Design review of the part built by this model. Coordinates are the model's own, in mm. A direction names the side the tool comes from. Give positions to 0.01 mm unless a question says otherwise; leave off trailing zeros. Order: outer loops, then holes, each group sorted by start corner. A loop starts at its lowest first (then second) coordinate and runs counter-clockwise, first axis right, second up. Notation, with made-up numbers: (-19, 10.25) -> (11, 10.25) arc R30 cw to (11, 48.25) -> close; hole circle Ø4 at (33, 60.25). An arc over 180 degrees is marked (long way). One line per item, written item: value.
from build123d import *

# Parameters (mm, degrees)
BOX_W             = 10
BOX_H             = 15
BOX_DEPTH         = 15
PAD_DEPTH         = 2
PAD_DEPTH_BACK    = 7.5
POCKET_DEPTH      = 6.4
POCKET001_DEPTH   = 2.5
PAD005_DEPTH      = 0.45
PAD005_DEPTH_BACK = 0.45
FILLET_R          = 0.5
FILLET008_R       = 0.2
FILLET009_R       = 0.2
FILLET010_R       = 0.5
SKETCH013_W       = 3
SKETCH013_H       = 1
PAD008_DEPTH      = 1
FILLET015_R       = 0.5
FILLET016_R       = 0.99


with BuildPart() as obj1:
    # Box → Box (new body)
    with BuildSketch(Plane(origin=(0, -9, 0), x_dir=(1, 0, 0), z_dir=(0, 0, 1))):
        with Locations((5, 7.5)):
            Rectangle(BOX_W, BOX_H)
    extrude(amount=BOX_DEPTH)


with BuildPart() as obj2:
    # Sketch (on DatumPlane) → Pad (new body, two sides)
    with BuildSketch(Plane.XY.offset(10)) as pad_sk:
        with BuildLine():
            ThreePointArc((5.5, 1.920538), (0, 2.6), (-5.5, 1.920538))
            Line((-5.5, 1.920538), (-3.616372, -5.586761))
            ThreePointArc((3.616372, -5.586761), (0, -5.14), (-3.616372, -5.586761))
            Line((3.616372, -5.586761), (5.5, 1.920538))
        make_face()
    extrude(amount=PAD_DEPTH)
    extrude(pad_sk.sketch, amount=-PAD_DEPTH_BACK)

    # Sketch001 (on Face5 of Pad) → Pocket (cut)
    with BuildSketch(Plane(origin=(0, 0, 2.5), x_dir=(1, 0, 0), z_dir=(0, 0, -1))):
        with BuildLine():
            ThreePointArc((-4.515394, -1.283614), (0, -1.8), (4.515394, -1.283614))
            Line((3.020793, 4.673197), (4.515394, -1.283614))
            ThreePointArc((-3.020793, 4.673197), (0, 4.34), (3.020793, 4.673197))
            Line((-4.515394, -1.283614), (-3.020793, 4.673197))
        make_face()
    extrude(amount=-POCKET_DEPTH, mode=Mode.SUBTRACT)

    # Sketch002 (on Face5 of Pocket) → Pocket001 (cut)
    with BuildSketch(Plane.XY.offset(12)):
        with BuildLine():
            ThreePointArc((4.283186, -2.929138), (0, -2.4), (-4.283186, -2.929138))
            Line((-4.283186, -2.929138), (-3.616372, -5.586761))
            ThreePointArc((3.616372, -5.586761), (0, -5.14), (-3.616372, -5.586761))
            Line((4.283186, -2.929138), (3.616372, -5.586761))
        make_face()
    extrude(amount=-POCKET001_DEPTH, mode=Mode.SUBTRACT)

    # Sketch008 (on DatumPlane) → Pad005 (join, two sides)
    with BuildSketch(Plane.XY.offset(7.95)) as pad005_sk:
        Polygon((-3.9, 2.260952), (-3.9, 4.3), (-3, 4.3), (-2.1, 4.3), (-2.1, 2.502222), align=None)
        Polygon((2.1, 2.502222), (2.1, 4.3), (3, 4.3), (3.9, 4.3), (3.9, 2.260952), align=None)
    extrude(amount=PAD005_DEPTH)
    extrude(pad005_sk.sketch, amount=-PAD005_DEPTH_BACK)

    # Fillet
    fillet_edges = [obj2.edges().sort_by_distance(p)[0] for p in [
        (0, -2.4, 12),
        (4.891593, -0.5043, 12),
        (0, 2.6, 12),
        (-4.891593, -0.5043, 12),
        (4.283186, -2.929138, 10.75),
        (5.5, 1.920538, 7.25),
        (-5.5, 1.920538, 7.25),
        (-4.283186, -2.929138, 10.75),
    ]]
    fillet(fillet_edges, radius=FILLET_R)

    # Fillet008
    fillet008_edges = [obj2.edges().sort_by_distance(p)[0] for p in [
        (-3.616372, -5.586761, 6),
        (3.616372, -5.586761, 6),
        (-4.496657, -2.078339, 2.5),
        (4.496657, -2.078339, 2.5),
    ]]
    fillet(fillet008_edges, radius=FILLET008_R)

    # Fillet009
    fillet009_edges = [obj2.edges().sort_by_distance(p)[0] for p in [
        (0, -4.34, 8.9),
        (-3.768094, -1.694791, 8.9),
        (0, 1.8, 8.9),
        (3.768094, -1.694791, 8.9),
        (4.515394, 1.283614, 5.7),
        (3.020793, -4.673197, 5.7),
        (-3.020793, -4.673197, 5.7),
        (-4.515394, 1.283614, 5.7),
    ]]
    fillet(fillet009_edges, radius=FILLET009_R)

    # Fillet010
    fillet010_edges = [obj2.edges().sort_by_distance(p)[0] for p in [
        (-3.002424, 2.399675, 8.4),
        (-3.002424, 2.399675, 7.5),
        (3.002424, 2.399675, 7.5),
        (3.002424, 2.399675, 8.4),
    ]]
    fillet(fillet010_edges, radius=FILLET010_R)

    # Sketch013 (on Face21 of Fillet010) → Pad008 (join)
    with BuildSketch(Plane(origin=(0, 0, 2.5), x_dir=(1, 0, 0), z_dir=(0, 0, -1))):
        with Locations((0, 3.921408)):
            Rectangle(SKETCH013_W, SKETCH013_H)
    extrude(amount=-PAD008_DEPTH)

    # Fillet015
    fillet015_edges = [obj2.edges().sort_by_distance(p)[0] for p in [
        (0, -4.34, 3.5),
    ]]
    fillet(fillet015_edges, radius=FILLET015_R)

    # Fillet016
    fillet016_edges = [obj2.edges().sort_by_distance(p)[0] for p in [
        (0, -3.421408, 3.5),
    ]]
    fillet(fillet016_edges, radius=FILLET016_R)

    # Cut: cut obj1
    add(obj1.part, mode=Mode.SUBTRACT)


solid = obj2.part
Item 1: Add section C-C on z = 10. Give the boundary of the cut face in (x, y), plus the area to 3 significant figures.
Returned:
outline: (-5.38, 1.43) -> (-4.4, -2.45) arc R0.5 ccw to (-3.81, -2.82) arc R17.6 cw to (0, -2.4) -> (0, 2.6) arc R22.6 ccw to (-5, 2.04) arc R0.5 ccw to start
area: 24.6 mm²
Item 2: Machinability: for faces 1 (the cylindrical face through (-1.444, -4.415, 5.557)), 2 (the cylindrical face through (-2.2, 1.68, 5.56)), 3 (the cylindrical face through (-4.737, -0.501, 11.857)), 4 (the flat face through (-3.9, 3, 8)), which of the approach directions +Z, -Z, +X, -X, +Y, -Y give a long, thin tool a straight path to every point of the face, cutting with its end or side? Answer none if there is none.
Returned:
face 1: none
face 2: -Z, +X
face 3: +Z, -X, -Y
face 4: +Z, -Z, -X, +Y
Item 3: To check wall thickness, follow line 1 along Z through (x, y) = (-3.55, 1.25); line 2 along Z through (x, y) = (-2.2, -4.25); line 3 along Y through (x, z) = (-2.8, 8). State the ranges of each line that lie inside material, in increasing order. Write a range as from..to.
Returned:
line 1: 8.9..12
line 2: 8.9..9.5
line 3: -5.41..-4.63, 1.6..4.3
Item 4: Add section B-B on y = 3.5. Give the boundary of the cut face in (x, z), plus the area to 3 significant figures.
Returned:
outline: (-3.9, 7.5) -> (-2.1, 7.5) -> (-2.1, 8.4) -> (-3.9, 8.4) -> close
area: 1.62 mm²
Item 5: Add section A-A on z = 7.75. Give the boundary of the cut face in (x, y).
Returned:
outline: (-5.38, 1.43) -> (-3.66, -5.39) arc R0.2 ccw to (-3.42, -5.54) arc R14.86 cw to (0, -5.14) -> (0, -4.34) arc R13.86 ccw to (-2.83, -4.63) arc R0.2 cw to (-3.07, -4.49) -> (-4.47, 1.09) arc R0.2 cw to (-4.31, 1.33) arc R20 cw to (0, 1.8) -> (0, 2.6) arc R22.6 ccw to (-2.1, 2.5) -> (-2.1, 4.3) -> (-3.9, 4.3) -> (-3.9, 2.26) arc R22.6 ccw to (-5, 2.04) arc R0.5 ccw to start
Item 6: Clearance check with flat-ended pins moving along their axes: P1, Ø3, axis at x = -1.5, z = 5, coming from the +Y side; P2, Ø1, axis at y = 3, z = 7.5, coming from the -X side; P3, Ø1.2, axis at x = -2.5, y = 3.5, coming from the +Z side. State where each tip first meets the part, or that it passes through.
Returned:
P1: y = 2.6
P2: x = -3.9
P3: z = 8.4
Item 7: Draft analysis for pull direction Y (two halves, no side actions). For faces 5 (the flat face through (-3.777, -1.661, 5.557)), 6 (the flat face through (-1.5, -4, 3)), 7 (the cylindrical face through (-1.7, -5.238, 6.049)), 8 (the flat face through (-3, 4, 8.4)), state which applies: pulls with the +Y half, pulls with the -Y half, needs draft (parallel to the pull), parting line crosses it, or undercut.
Returned:
face 5: undercut
face 6: undercut
face 7: pulls with the -Y half
face 8: needs draft
